Autodesk Inventor part; units mm, degrees
ref_plane "YZ Plane" through (0, 0, 0) normal (1, 0, 0) x (0, 1, 0)
ref_plane "XZ Plane" through (0, 0, 0) normal (0, 1, 0) x (-1, 0, 0)
ref_plane "XY Plane" through (0, 0, 0) normal (0, 0, 1) x (1, 0, 0)
sketch "Sketch1" plane through (0, 0, 0) normal (0, 1, 0) x (-1, 0, 0)
  line L0 (0, 0) -> (90, 0)
  line L1 (90, 0) -> (90, -112.5)
  line L2 (90, -112.5) -> (0, -112.5)
  line L3 (0, -112.5) -> (0, 0)
  dimension "d0" = 90
  dimension "d1" = 112.5
extrude "Extrusion1" add sketch "Sketch1" along normal blind 3
sketch "Sketch3" plane through (-90, 0, 0) normal (0, 0, 1) x (1, 0, 0)
  line L0 (90, 0) -> (0, 0)
  line L1 (90, 3) -> (0, 3)
  line L2 (0, 0) -> (75, 0)
  line L3 (75, 0) -> (75, 3)
  line L4 (75, 3) -> (0, 3)
  line L5 (0, 3) -> (0, 0)
  line L6 (90, 0) -> (90, 3)
  point P0 (0, 3)
  dimension "d5" = 15
extrude "Extrusion2" add sketch "Sketch3" along normal blind 18 contours L0 L5 L1 L3
sketch "Sketch4" plane through (0, 3, 0) normal (0, 1, 0) x (1, 0, 0)
  line L0 (-6, 128.5084) -> (-6, -27.8518) construction
  line L1 (-118.0415, 106.5) -> (21.4799, 106.5) construction
  line L2 (-84, 125.301) -> (-84, -43.3542) construction
  line L3 (-90, 112.5) -> (-90, -18)
  line L4 (0, 112.5) -> (-90, 112.5)
  line L5 (0, 0) -> (0, 112.5)
  line L6 (-35.7185, 6) -> (24.9546, 6) construction
  line L7 (-15, 0) -> (0, 0)
  point P0 (-7.5, 6)
  point P1 (-6, 106.5)
  point P2 (-45, 106.5)
  point P3 (-84, 106.5)
  point P4 (-84, 72.5)
  point P5 (-84, 38.5)
  dimension "d8" = 6
  dimension "d9" = 6
  dimension "d10" = 6
  dimension "d11" = 6
  dimension "d12" = 7.5
  dimension "d13" = 39
  dimension "d14" = 34
  dimension "d15" = 34
hole "Hole1" at (-7.5, 3, -6) at (-6, 3, -106.5) at (-45, 3, -106.5) at (-84, 3, -106.5) at (-84, 3, -72.5) at (-84, 3, -38.5) direction (0, -1, 0) diameter 3.2 end through all
properties part number "Gas Side Top Cover"
Verification items for the finished model (mm, model axes). A direction names the side the tool comes from. Coordinates: 2 decimals unless noted, no trailing zeros. Loops run counter-clockwise (first coordinate to the right, second up) from the corner with the lowest first, then second, coordinate; pieces in that order, holes last. Notation, with made-up numbers: (80.25, 35) -> (135.25, 35) arc R18 ccw to (135.25, 65) -> close; hole circle Ø1 at (42.25, 6.5). An arc over 180 degrees is marked (long way). Answer in a Markdown table with one row per item.
1) Section check C-C (y = 1.5). Record the cut outline in (x, z), and give its area (3 significant figures).
The answers:
| item | result |
|---|---|
| outline | (-90, -112.5) -> (0, -112.5) -> (0, 0) -> (-15, 0) -> (-15, 18) -> (-90, 18) -> close; hole circle Ø3.2 at (-84, -106.5); hole circle Ø3.2 at (-84, -72.5); hole circle Ø3.2 at (-84, -38.5); hole circle Ø3.2 at (-45, -106.5); hole circle Ø3.2 at (-7.5, -6); hole circle Ø3.2 at (-6, -106.5) |
| area | 11,400 mm2 |
2) Section check D-D (x = -11.5). Record the cut outline in (y, z), and give its area (4 significant figures).
The answers:
| item | result |
|---|---|
| outline | (0, -112.5) -> (3, -112.5) -> (3, 0) -> (0, 0) -> close |
| area | 337.5 mm2 |
3) Access from +Z, -Z, +X, -X, +Y, -Y to the whole of each face (thin tool, end or side, straight path). Record for faces 5 (the face through (-15, 1, 9)), 6 (the face through (-84.07, 1.48, -108.1)).
The answers:
| item | result |
|---|---|
| face 5 | +Z, +X, +Y, -Y |
| face 6 | +Y, -Y |
4) Draft check along Z on faces 1 (the face through (-44, 0, -46)), 2 (the face through (-85.586, 1.479, -38.708)), 3 (the face through (-6.07, 1.48, -108.1)), 4 (the face through (-53, 2, 18)). Enter one of: released by +Z, released by -Z, zero draft, split by the parting line, or undercut.
The answers:
| item | result |
|---|---|
| face 1 | zero draft |
| face 2 | undercut |
| face 3 | undercut |
| face 4 | released by +Z |
5) Section check A-A (z = -72.5). Record the cut outline in (x, y), and give its area (3 significant figures).
The answers:
| item | result |
|---|---|
| outline | (-90, 0) -> (-85.6, 0) -> (-85.6, 3) -> (-90, 3) -> close; (-82.4, 0) -> (0, 0) -> (0, 3) -> (-82.4, 3) -> close |
| area | 260 mm2 |
6) Section check B-B (x = -84). Record the cut outline in (y, z), and give its area (3 significant figures).
The answers:
| item | result |
|---|---|
| outline | (0, -112.5) -> (3, -112.5) -> (3, -108.1) -> (0, -108.1) -> close; (0, -104.9) -> (3, -104.9) -> (3, -74.1) -> (0, -74.1) -> close; (0, -70.9) -> (3, -70.9) -> (3, -40.1) -> (0, -40.1) -> close; (0, -36.9) -> (3, -36.9) -> (3, 18) -> (0, 18) -> close |
| area | 363 mm2 |
7) Scan lines: line 1 along Z through (x, y) = (-84, 1.5); line 2 along X through (y, z) = (1, -106.5); line 3 along Z through (x, y) = (-45, 1.1). Record each from-to range of solid material in increasing order. Write a range as from..to.
The answers:
| item | result |
|---|---|
| line 1 | z = -112.5..-108.1, -104.9..-74.1, -70.9..-40.1, -36.9..18 |
| line 2 | x = -90..-85.6, -82.4..-46.6, -43.4..-7.6, -4.4..0 |
| line 3 | z = -112.5..-108.1, -104.9..18 |
8) Depth check by flat-ended pin: P1, Ø2.5, axis at x = -84, z = -38.5, coming from the -Y side; P2, Ø1.5, axis at y = 1.5, z = 12, coming from the +X side; P3, Ø0.9, axis at x = -11, y = 1.5, coming from the +Z side. Enter the tip coordinate at first touch or a pass-through.
The answers:
| item | result |
|---|---|
| P1 | passes through |
| P2 | stops at x = -15 |
| P3 | stops at z = 0 |
